Here's how the part is built. I have some questions about the finished solid (model axes, mm). A direction names the side the tool comes from. Round coordinates to 2 decimals unless told otherwise and drop trailing zeros. Write each loop counter-clockwise with the first axis right and the second up, starting at its lowest first coordinate (ties: lowest second). Pieces come first, ordered by that corner, then holes. Notation, with made-up numbers: (-36.75, -15.75) - (-20.75, -15.75) arc R20 ccw to (-20.75, 12.25) - close; hole circle Ø7 at (21.5, -20). An arc over 180 degrees is marked (long way). Write item = value, one per line. Start each with the question number.
Item 1: If we section it at B-B (y = 257): Please give me the cut outline in (x, z), and give its area (3 significant figures).
Item 2: If I drill on line 1 along X through (y, z) = (149, -1); line 2 along Z through (x, y) = (56, 400); line 3 along Y through (x, z) = (57, -0.75), over which ranges is the centre line in solid material (lowest first)? Write a range as [from, to].
Item 3: If we section it at C-C (x = 40): Please give me the cut outline in (y, z), and give its area (3 significant figures).
Item 4: If we section it at A-A (z = 5.25): Please give me the cut outline in (x, y).
Item 5: For P1, Ø12, axis at y = 287, z = 1, coming from the -X side; P2, Ø3, axis at x = 53.5, z = -4, coming from the -Y side; P3, Ø5, axis at x = 25.5, z = 2.5, coming from the +Y side; P4, Ø4, axis at y = 46, z = -4, coming from the +X side, each with a flat end and sliding along its axis, tell me the tip position at first contact or that it passes through.
Item 6: Which directions (+Z, -Z, +X, -X, +Y, -Y) give clear straight access to the entire face, cutting with the end or side of a thin tool? Please do faces 1 (the face through (-2.222, 187.59, 10.006)), 2 (the face through (90, 395, 8)).
Item 7: Thinking about a two-plate mould opening in Z: for faces 3 (the face through (60.42, 391.654, -2.628)), 4 (the face through (5, 0, 8)), 5 (the face through (8.346, 187.59, -2.628)), 6 (the face through (60.42, 390.532, 3.926)), which applies, pulls with the +Z half, pulls with the -Z half, needs draft (parallel to the pull), parting line crosses it, or undercut?
```python
from build123d import *

# Parameters (mm, degrees)
ESBO_O2_R             = 10.25
ESBO_O2_R_2           = 8.75
FURO_ROSCADO_DE_M51_D = 4.2
PADR_O_LINEAR1_COUNT  = 4
PADR_O_LINEAR1_PITCH  = 45


with BuildPart() as part:
    # Varredura1: sweep along a path in Esboço1
    with BuildLine(Plane.XY) as varredura1_path:
        Line((0, 0), (0, 370))
        ThreePointArc((0, 370), (8.786796564, 391.213203436), (30, 400))
        Line((30, 400), (90, 400))
    # Esboço2 → Varredura1 (sweep)
    with BuildSketch(Plane(origin=(0, 0, 0), x_dir=(1, 0, 0), z_dir=(0, 1, 0))):
        Circle(ESBO_O2_R)
        Circle(ESBO_O2_R_2, mode=Mode.SUBTRACT)
    sweep(path=varredura1_path.line)

    # Furo roscado de M51 (through all)
    with Locations(Plane.XY.offset(11)):
        with Locations((0, 20)):
            furo_roscado_de_m51 = Hole(FURO_ROSCADO_DE_M51_D / 2)

    # Padrão linear1: Furo roscado de M51 ×4
    with Locations(*[(0, i * PADR_O_LINEAR1_PITCH, 0) for i in range(1, PADR_O_LINEAR1_COUNT)]):
        add(furo_roscado_de_m51, mode=Mode.SUBTRACT)


solid = part.part
```
Reply:
q1.outline = circle Ø20.5 at (0, 0); hole circle Ø17.5 at (0, 0)
q1.area = 89.5 mm2
q2.line_1 = [-10.2, -8.69], [8.69, 10.2]
q2.line_2 = [-10.25, -8.75], [8.75, 10.25]
q2.line_3 = [389.78, 391.28], [408.72, 410.22]
q3.outline = circle Ø20.5 at (400, 0); hole circle Ø17.5 at (400, 0)
q3.area = 89.5 mm2
q4.outline = (-8.8, 0) - (-7, 0) - (-7, 370) arc R37 cw to (30, 407) - (90, 407) - (90, 408.8) - (30, 408.8) arc R38.8 ccw to (-8.8, 370) - close; (7, 0) - (8.8, 0) - (8.8, 370) arc R21.2 cw to (30, 391.2) - (90, 391.2) - (90, 393) - (30, 393) arc R23 ccw to (7, 370) - close
q5.P1 = -10.25
q5.P2 = 390.06
q5.P3 = 410.13
q5.P4 = 10.05
q6.face_1 = -Y
q6.face_2 = +Z, -Z, +X, +Y, -Y
q7.face_3 = undercut
q7.face_4 = needs draft
q7.face_5 = undercut
q7.face_6 = parting line crosses it
